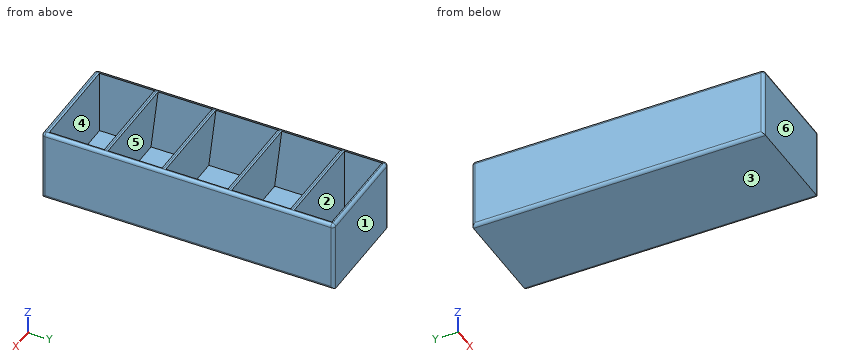
from build123d import *

# Parameters (mm, degrees)
F0_W        = 65
F0_H        = 182
F1_DEPTH    = 45
F2_W        = 60
F2_H        = 175
F3_DEPTH    = 40
F5_DEPTH    = 65
F6_R        = 2
F7_T1_DEPTH = 60


# Not quite as in the source:
# - a fillet or chamfer that OpenCascade refuses, or shapes differently, is made with other operations: its cross-section is extruded or revolved along the edge and cut away or added


with BuildPart() as f1:
    # F0 (on Top) → F1 (new body)
    with BuildSketch(Plane.XY):
        Rectangle(F0_W, F0_H)
    extrude(amount=F1_DEPTH)

    # F2 (on face) → F3 (cut)
    with BuildSketch(Plane.XY.offset(45)):
        Rectangle(F2_W, F2_H)
    extrude(amount=-F3_DEPTH, mode=Mode.SUBTRACT)

    # F4 (on face) → F5 (join)
    with BuildSketch(Plane.YZ.offset(32.5)):
        Polygon((-51, 45), (-54, 45), (-59, 0), (-56, 0), align=None)
        Polygon((-15, 45), (-18, 45), (-23, 0), (-20, 0), align=None)
        Polygon((26, 45), (23, 45), (18, 0), (21, 0), align=None)
        Polygon((65, 45), (62, 45), (57, 0), (65, 0), align=None)
    extrude(amount=-F5_DEPTH)

    # F6
    f6_edges = [f1.edges().sort_by_distance(p)[0] for p in [
        (-32.5, 0, 0),
        (-32.5, 91, 22.5),
        (-32.5, 0, 45),
        (-32.5, -91, 22.5),
        (32.5, 0, 0),
        (32.5, -91, 22.5),
        (32.5, 0, 45),
        (32.5, 91, 22.5),
        (0, -91, 45),
        (0, 91, 45),
    ]]
    fillet(f6_edges, radius=F6_R)

    # F7: fillet of radius 2 on 5 edges, made by hand

    # F7_s2 → F7_t1 (cut)
    with BuildSketch(Plane.YZ.offset(-30)):
        with BuildLine():
            ThreePointArc((-52.2099144137, 45), (-53.5437573385, 44.4902560358), (-54.1976818831, 43.2208630521))
            Line((-54.1976818831, 43.2208630521), (-54, 45))
            Line((-54, 45), (-52.2099144137, 45))
        make_face()
        with BuildLine():
            ThreePointArc((-16.2099144137, 45), (-17.5437573385, 44.4902560358), (-18.1976818831, 43.2208630521))
            Line((-18.1976818831, 43.2208630521), (-18, 45))
            Line((-18, 45), (-16.2099144137, 45))
        make_face()
        with BuildLine():
            ThreePointArc((24.7900855863, 45), (23.4562426615, 44.4902560358), (22.8023181169, 43.2208630521))
            Line((22.8023181169, 43.2208630521), (23, 45))
            Line((23, 45), (24.7900855863, 45))
        make_face()
        with BuildLine():
            ThreePointArc((63.7900855863, 45), (62.4562426615, 44.4902560358), (61.8023181169, 43.2208630521))
            Line((61.8023181169, 43.2208630521), (62, 45))
            Line((62, 45), (63.7900855863, 45))
        make_face()
        with BuildLine():
            ThreePointArc((89.5, 45), (88.0857864376, 44.4142135624), (87.5, 43))
            Line((87.5, 43), (87.5, 45))
            Line((87.5, 45), (89.5, 45))
        make_face()
    extrude(amount=F7_T1_DEPTH, mode=Mode.SUBTRACT)


solid = f1.part
Design review of the part built by this model. Coordinates are the model's own, in mm. Face numbers are marked on the shaded views. A direction names the side the tool comes from. Give positions to 0.01 mm unless a question says otherwise; leave off trailing zeros. Write each loop counter-clockwise with the first axis right and the second up, starting at its lowest first coordinate (ties: lowest second). Pieces come first, ordered by that corner, then holes. Notation, with made-up numbers: M 70,-36.75 L 129,-36.75 A25 ccw 129,-24.75 Z; hole C 46.5,-38.5 d9. An arc over 180 degrees is marked long. Answer as a JSON object with one key per item and string values. Group by question number.
1) We need section B-B (y = -9.5). Give the boundary of the cut face in (x, z), and give its area (3 significant figures).
2) Clearance check with flat-ended pins moving along their axes: pin 1 Ø25 at (x, y) = (9.5, 80) entering from +Z; pin 2 Ø8.5 at (x, y) = (-2, -67) entering from +Z. State where each tip first meets the part, or that it passes through.
3) We need section A-A (z = 40.5). Give the boundary of the cut face in (x, y), and give its area (3 significant figures).
4) Mouldability with a two-part tool opening along Y and no side actions: class the marked faces 1, 2 and 3 as released by +Y, released by -Y, zero draft, split by the parting line, or undercut.
5) For line 1 along X through (y, z) = (-65, 24.5); line 2 along Y through (x, z) = (-27, 23.5); line 3 along Y through (x, z) = (0, 5.5), list the stretches that pass through material, from the lowest coordinate up.
6) Tool access review of the marked faces 4, 5 and 6: name each direction out of +Z, -Z, +X, -X, +Y, -Y from which nothing blocks a thin tool from reaching the whole face with its end or side.
7) We need section D-D (z = 17.5). Give the boundary of the cut face in (x, y), and give its area (3 significant figures).
Answer key:
{
 "1": {"outline": "M -32.5,2 A2 ccw -30.5,0 L 30.5,0 A2 ccw 32.5,2 L 32.5,43 A2 ccw 30.5,45 L 30,45 L 30,5 L -30,5 L -30,45 L -30.5,45 A2 ccw -32.5,43 Z", "area": "522 mm²"},
 "2": {"pin 1": "stops at z = 44.98", "pin 2": "stops at z = 5"},
 "3": {"outline": "M -32.5,-89 A2 ccw -30.5,-91 L 30.5,-91 A2 ccw 32.5,-89 L 32.5,89 A2 ccw 30.5,91 L -30.5,91 A2 ccw -32.5,89 Z; hole M -30,-87.5 L 30,-87.5 L 30,-54.5 L -30,-54.5 Z; hole M -30,-51.5 L 30,-51.5 L 30,-18.5 L -30,-18.5 Z; hole M -30,-15.5 L 30,-15.5 L 30,22.5 L -30,22.5 Z; hole M -30,25.5 L 30,25.5 L 30,61.5 L -30,61.5 Z; hole M -30,65 L 30,65 L 30,87.5 L -30,87.5 Z", "area": "2,080 mm²"},
 "4": {"face 1": "released by +Y", "face 2": "undercut", "face 3": "zero draft"},
 "5": {"line 1": "x = -32.5 to -30, 30 to 32.5", "line 2": "y = -91 to -87.5, -56.39 to -53.39, -20.39 to -17.39, 20.61 to 23.61, 59.61 to 65, 87.5 to 91", "line 3": "y = -91 to -87.5, -58.39 to -55.39, -22.39 to -19.39, 18.61 to 21.61, 57.61 to 65, 87.5 to 91"},
 "6": {"face 4": "+Z", "face 5": "none", "face 6": "+Z, -Z, +X, -X, -Y"},
 "7": {"outline": "M -32.5,-89 A2 ccw -30.5,-91 L 30.5,-91 A2 ccw 32.5,-89 L 32.5,89 A2 ccw 30.5,91 L -30.5,91 A2 ccw -32.5,89 Z; hole M -30,-87.5 L 30,-87.5 L 30,-57.06 L -30,-57.06 Z; hole M -30,-54.06 L 30,-54.06 L 30,-21.06 L -30,-21.06 Z; hole M -30,-18.06 L 30,-18.06 L 30,19.94 L -30,19.94 Z; hole M -30,22.94 L 30,22.94 L 30,58.94 L -30,58.94 Z; hole M -30,65 L 30,65 L 30,87.5 L -30,87.5 Z", "area": "2,230 mm²"}
}
